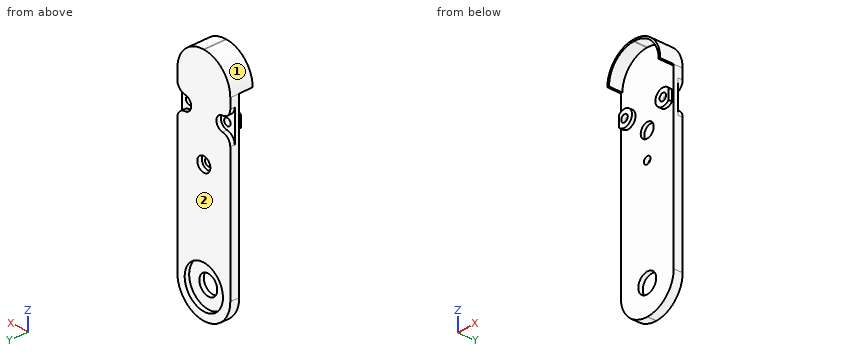
from build123d import *

# Parameters (mm, degrees)
BOSS_EXTRUDE1_DEPTH = 10
SKETCH2_R           = 23.5
CUT_EXTRUDE1_DEPTH  = 5
SKETCH3_R           = 11
CUT_EXTRUDE2_DEPTH  = 135.094183319
SKETCH22_R          = 8
CUT_EXTRUDE15_DEPTH = 4
SKETCH23_R          = 4
BOSS_EXTRUDE6_DEPTH = 4
SKETCH24_R          = 4
CUT_EXTRUDE16_DEPTH = 135.373546504
BOSS_EXTRUDE7_START = 15
BOSS_EXTRUDE7_DEPTH = 15
SKETCH26_R          = 8
CUT_EXTRUDE17_DEPTH = 5
FILLET1_R           = 10
FILLET2_R           = 10


with BuildPart() as part:
    # Sketch1 → Boss-Extrude1 (new body)
    with BuildSketch(Plane(origin=(0, 0, 0), x_dir=(1, 0, 0), z_dir=(0, 1, 0))):
        with BuildLine():
            Line((0, 130), (0.5, 130))
            ThreePointArc((0.5, 130), (23.127416998, 120.627416998), (32.5, 98))
            Line((32.5, 98), (32.5, -98))
            ThreePointArc((32.5, -98), (23.127416998, -120.627416998), (0.5, -130))
            Line((0.5, -130), (-0.5, -130))
            ThreePointArc((-0.5, -130), (-23.127416998, -120.627416998), (-32.5, -98))
            Line((-32.5, -98), (-32.5, 97.5))
            ThreePointArc((-32.5, 97.5), (-22.980970389, 120.480970389), (0, 130))
        make_face()
    extrude(amount=BOSS_EXTRUDE1_DEPTH)

    # Sketch2 → Cut-Extrude1 (cut)
    with BuildSketch(Plane(origin=(0, 10, 0), x_dir=(1, 0, 0), z_dir=(0, 1, 0))):
        with Locations(Location((0, 97.5, 0), (0, 0, 270))):
            Circle(SKETCH2_R)
    extrude(amount=-CUT_EXTRUDE1_DEPTH, mode=Mode.SUBTRACT)

    # Sketch3 → Cut-Extrude2 (cut, through all)
    with BuildSketch(Plane(origin=(0, 5, 0), x_dir=(1, 0, 0), z_dir=(0, 1, 0))):
        with Locations(Location((0, 97.5, 0), (0, 0, 270))):
            Circle(SKETCH3_R)
    extrude(amount=-CUT_EXTRUDE2_DEPTH, mode=Mode.SUBTRACT)

    # Sketch22 → Cut-Extrude15 (cut)
    with BuildSketch(Plane.XZ):
        with Locations(Location((0, 48.75, 0), (0, 0, 270))):
            Circle(SKETCH22_R)
    extrude(amount=-CUT_EXTRUDE15_DEPTH, mode=Mode.SUBTRACT)

    # Sketch23 → Boss-Extrude6 (add)
    # profile 1 of 2: a face of its own
    with BuildSketch(Plane.XZ):
        with BuildLine():
            Line((-30.5, 74.616516124), (-30.5, 62.993052049))
            ThreePointArc((-30.5, 62.993052049), (-14.401855723, 68.804784086), (-30.5, 74.616516124))
        make_face()
        with Locations(Location((-23.5, 68.804784086, 0), (0, 0, 270))):
            Circle(SKETCH23_R, mode=Mode.SUBTRACT)
    # profile 2 of 2: a face of its own
    with BuildSketch(Plane.XZ):
        with BuildLine():
            Line((30.5, 74.616516124), (30.5, 62.993052049))
            ThreePointArc((30.5, 62.993052049), (14.401855723, 68.804784086), (30.5, 74.616516124))
        make_face()
        with Locations(Location((23.5, 68.804784086, 0), (0, 0, 90))):
            Circle(SKETCH23_R, mode=Mode.SUBTRACT)
    extrude(amount=BOSS_EXTRUDE6_DEPTH)

    # Sketch24 → Cut-Extrude16 (cut, through all)
    with BuildSketch(Plane.XZ):
        with Locations(Location((0, 20, 0), (0, 0, 270))):
            Circle(SKETCH24_R)
        with Locations(Location((-23.5, 68.804784086, 0), (0, 0, 270))):
            Circle(SKETCH24_R)
        with Locations(Location((23.5, 68.804784086, 0), (0, 0, 90))):
            Circle(SKETCH24_R)
    extrude(amount=-CUT_EXTRUDE16_DEPTH, mode=Mode.SUBTRACT)

    # Sketch25 → Boss-Extrude7 (add)
    with BuildSketch(Plane.XZ.offset(BOSS_EXTRUDE7_START)):
        with BuildLine():
            Line((-32.5, 98), (-30.5, 98))
            ThreePointArc((-30.5, 98), (-21.713203436, 119.213203436), (-0.5, 128))
            Line((-0.5, 128), (0.5, 128))
            ThreePointArc((0.5, 128), (21.713203436, 119.213203436), (30.5, 98))
            Line((30.5, 98), (32.5, 98))
            ThreePointArc((32.5, 98), (23.127416998, 120.627416998), (0.5, 130))
            Line((0.5, 130), (-0.5, 130))
            ThreePointArc((-0.5, 130), (-23.127416998, 120.627416998), (-32.5, 98))
        make_face()
    extrude(amount=-BOSS_EXTRUDE7_DEPTH)

    # Sketch26 → Cut-Extrude17 (cut)
    with BuildSketch(Plane(origin=(0, 10, 0), x_dir=(1, 0, 0), z_dir=(0, 1, 0))):
        with Locations(Location((0, -20, 0), (0, 0, 270))):
            Circle(SKETCH26_R)
        with BuildLine():
            Line((-23.5, -60.804784086), (-32.5, -60.804784086))
            Line((-32.5, -60.804784086), (-32.5, -76.804784086))
            Line((-32.5, -76.804784086), (-23.5, -76.804784086))
            ThreePointArc((-23.5, -76.804784086), (-15.5, -68.804784086), (-23.5, -60.804784086))
        make_face()
        with BuildLine():
            Line((23.5, -60.804784086), (32.5, -60.804784086))
            Line((32.5, -60.804784086), (32.5, -76.804784086))
            Line((32.5, -76.804784086), (23.5, -76.804784086))
            ThreePointArc((23.5, -76.804784086), (15.5, -68.804784086), (23.5, -60.804784086))
        make_face()
    extrude(amount=-CUT_EXTRUDE17_DEPTH, mode=Mode.SUBTRACT)

    # Fillet1
    # the kernel refuses this fillet: 10 mm, written as the material it takes off along each edge
    with BuildSketch(Plane(origin=(-32.5, 34.930501889, 76.804784086), x_dir=(0, 0, 1), z_dir=(0, -1, 0))) as fillet1_piece_1:
        with BuildLine():
            CenterArc((9.972200756, -10), FILLET1_R, 90, 86.815261463)
            Line((-0.01235522, -9.444444444), (-1.010810817, -9.388888889))
            ThreePointArc((-1.010810817, -9.388888889), (-1, -9), (-1, 0))
            Line((-1, 0), (0, 1))
            Line((0, 1), (9.972200756, 1))
            Line((9.972200756, 1), (9.972200756, 0))
        make_face()
    extrude(amount=29.930501889, mode=Mode.SUBTRACT)
    with BuildSketch(Plane(origin=(-32.5, 34.930501889, 60.804784086), x_dir=(0, 0, -1), z_dir=(0, -1, 0))) as fillet1_piece_2:
        with BuildLine():
            CenterArc((9.972200756, 10), FILLET1_R, 183.184738537, 86.815261463)
            Line((-0.01235522, 9.444444444), (-1.010810817, 9.388888889))
            ThreePointArc((-1.010810817, 9.388888889), (-1, 9), (-1, 0))
            Line((-1, 0), (0, -1))
            Line((0, -1), (9.972200756, -1))
            Line((9.972200756, -1), (9.972200756, 0))
        make_face()
    extrude(amount=29.930501889, mode=Mode.SUBTRACT)

    # Fillet2
    # the kernel refuses this fillet: 10 mm, written as the material it takes off along each edge
    with BuildSketch(Plane(origin=(32.5, 34.930501889, 76.804784086), x_dir=(0, 0, 1), z_dir=(0, -1, 0))) as fillet2_piece_1:
        with BuildLine():
            CenterArc((9.972200756, 10), FILLET2_R, 183.184738537, 86.815261463)
            Line((-0.01235522, 9.444444444), (-1.010810817, 9.388888889))
            ThreePointArc((-1.010810817, 9.388888889), (-1, 9), (-1, 0))
            Line((-1, 0), (0, -1))
            Line((0, -1), (9.972200756, -1))
            Line((9.972200756, -1), (9.972200756, 0))
        make_face()
    extrude(amount=29.930501889, mode=Mode.SUBTRACT)
    with BuildSketch(Plane(origin=(32.5, 34.930501889, 60.804784086), x_dir=(0, 0, -1), z_dir=(0, -1, 0))) as fillet2_piece_2:
        with BuildLine():
            CenterArc((9.972200756, -10), FILLET2_R, 90, 86.815261463)
            Line((-0.01235522, -9.444444444), (-1.010810817, -9.388888889))
            ThreePointArc((-1.010810817, -9.388888889), (-1, -9), (-1, 0))
            Line((-1, 0), (0, 1))
            Line((0, 1), (9.972200756, 1))
            Line((9.972200756, 1), (9.972200756, 0))
        make_face()
    extrude(amount=29.930501889, mode=Mode.SUBTRACT)


solid = part.part
Design review of the part built by this model. Coordinates are the model's own, in mm. Face numbers are marked on the shaded views. Give positions to 0.01 mm unless a question says otherwise; leave off trailing zeros. Write each loop counter-clockwise with the first axis right and the second up, starting at its lowest first coordinate (ties: lowest second). Pieces come first, ordered by that corner, then holes. Notation, with made-up numbers: M 18.5,55 L 66.5,55 A22 ccw 66.5,69 Z; hole C 56.5,21.25 d7. An arc over 180 degrees is marked long. Return JSON: item names as keys, results as strings. Group by question number.
Item 1: Clearance check with flat-ended pins moving along their axes: pin 1 Ø1.5 at (x, y) = (3, -3) entering from +Z; pin 2 Ø8 at (x, y) = (-13.5, -5) entering from -Z; pin 3 Ø1.6 at (x, y) = (-31.5, -8) entering from -Z; pin 4 Ø4 at (y, z) = (-2.5, -97) entering from -X. State where each tip first meets the part, or that it passes through.
Item 2: The part is to be moulded in two halves that separate along Z. For the marked faces 1 and 2, say which applies: pulls with the +Z half, pulls with the -Z half, needs draft (parallel to the pull), parting line crosses it, or undercut.
Item 3: Wall thickness on line 1 along X through (y, z) = (1.55, 20); line 2 along Y through (x, z) = (5.5, -111); line 3 along Y through (x, z) = (20.5, 73): over which ranges is each line inside the solid? List them lowest first.
Item 4: Take a section at C-C (z = -43.5). Give the boundary of the cut face in (x, y).
Item 5: Take a section at B-B (y = -7). Give the boundary of the cut face in (x, z).
Item 6: Take a section at A-A (z = 20). Give the boundary of the cut face in (x, y).
Return value:
{
 "1": {"pin 1": "stops at z = 129.95", "pin 2": "stops at z = 62.08", "pin 3": "stops at z = 98", "pin 4": "passes through"},
 "2": {"face 1": "pulls with the +Z half", "face 2": "needs draft"},
 "3": {"line 1": "x = -32.5 to -4, 4 to 32.5", "line 2": "y = 0 to 5", "line 3": "y = -4 to 5"},
 "4": {"outline": "M -32.5,0 L 32.5,0 L 32.5,10 L -32.5,10 Z"},
 "5": {"outline": "M -32.5,98 L -30.5,98 A30 cw -0.5,128 L 0.5,128 A30 cw 30.5,98 L 32.5,98 A32 ccw 0.5,130 L -0.5,130 A32 ccw Z"},
 "6": {"outline": "M -32.5,0 L -4,0 L -4,5 L -8,5 L -8,10 L -32.5,10 Z; M 4,0 L 32.5,0 L 32.5,10 L 8,10 L 8,5 L 4,5 Z"}
}
